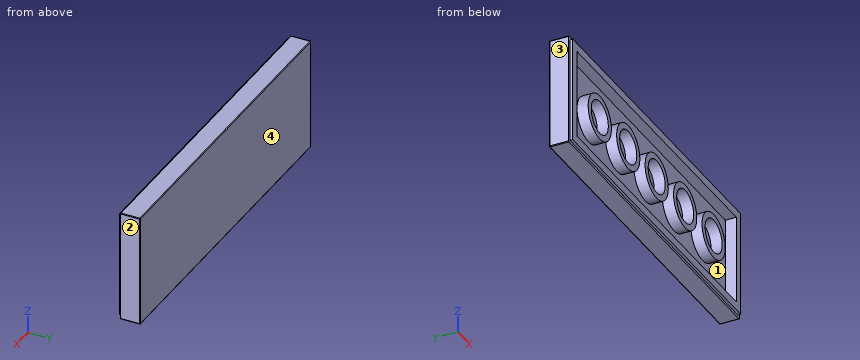
Autodesk Inventor part; units mm, degrees
ref_plane "YZ Plane" through (0, 0, 0) normal (1, 0, 0) x (0, 1, 0)
ref_plane "XZ Plane" through (0, 0, 0) normal (0, 1, 0) x (-1, 0, 0)
ref_plane "XY Plane" through (0, 0, 0) normal (0, 0, 1) x (1, 0, 0)
sketch "Sketch2" plane through (0, 0, 0) normal (0, 1, 0) x (-1, 0, 0)
  line L0 (-24, 8) -> (24, 8)
  line L1 (24, 8) -> (24, -8)
  line L2 (24, -8) -> (-24, -8)
  line L3 (-24, -8) -> (-24, 8)
  point P0 (0, 0)
  point P1 (0, 8)
  point P2 (-24, 0)
  dimension "d0" = 48
  dimension "d1" = 16
extrude "Extrusion1" add sketch "Sketch2" along normal blind 3.2
sketch "Sketch3" plane through (0, 0, 0) normal (0, -1, 0) x (1, 0, 0)
  line L0 (-24, 8) -> (-24, -8)
  line L1 (-22.4, 6.4) -> (22.4, 6.4)
  line L2 (22.4, 6.4) -> (22.4, -6.4)
  line L3 (22.4, -6.4) -> (-22.4, -6.4)
  line L4 (-22.4, -6.4) -> (-22.4, 6.4)
  circle A0 centre (-16, 0) radius 3.2569
  circle A1 centre (-16, 0) radius 2.4
  line L5 (-24, -8) -> (24, -8)
  circle A2 centre (0, 0) radius 1.6
  line L6 (24, -8) -> (24, 8)
  line L7 (-12, 0) -> (-4, 0) construction
  line L8 (-4, 0) -> (4, 0) construction
  line L9 (4, 0) -> (12, 0) construction
  circle A3 centre (-20, 4) radius 2.4 construction
  circle A4 centre (-20, -4) radius 2.4 construction
  circle A5 centre (20, -4) radius 2.4 construction
  circle A6 centre (20, 4) radius 2.4 construction
  line L10 (24, 8) -> (-24, 8)
  line L11 (-23.6, 7.6) -> (23.6, 7.6)
  line L12 (23.6, 7.6) -> (23.6, -7.6)
  line L13 (23.6, -7.6) -> (-23.6, -7.6)
  line L14 (-23.6, -7.6) -> (-23.6, 7.6)
  point P0 (-22.4, 0)
  point P1 (0, 6.4)
  point P2 (0, 0)
  point P3 (0, 7.6)
  point P4 (-23.6, 0)
  dimension "d61" = 4.8
  dimension "d75" = 8
  dimension "d76" = 8
  dimension "d86" = 3.2
  dimension "d92" = 8
  dimension "d98" = 40
  dimension "d99" = 8
  dimension "d102" = 0.4
  dimension "d103" = 0.4
extrude "Extrusion2" cut sketch "Sketch3" against normal blind 1.6 contours L1 L2 L3 L4 | A0 | A1 | A2
extrude "Extrusion7" cut sketch "Sketch3" against normal blind 0.4 contours L10 L6 L5 L0
extrude "Extrusion6" add sketch "Sketch3" against normal up to next contours A0
pattern_linear "Rectangular Pattern3" count 5 spacing 8 along (1, 0, 0) of "Extrusion6"
fillet "Fillet1" radius 0.1 8 edges at (-24, 1.8, 8) (0, 3.2, 8) (-24, 3.2, 0) (0, 3.2, -8) (24, 3.2, 0) (24, 1.8, 8) (24, 1.8, -8) (-24, 1.8, -8)
sketch "Skizze10" plane through (0, 3.2, 0) normal (0, 1, 0) x (1, 0, 0)
  line L0 (-21.913, 4.8) -> (21.913, 4.8) construction
  line L1 (21.913, 4.8) -> (21.913, -4.8) construction
  line L2 (21.913, -4.8) -> (-21.913, -4.8) construction
  line L3 (-21.913, -4.8) -> (-21.913, 4.8) construction
  line L4 (23.9, 8) -> (-23.9, 8)
  line L5 (-23.9, -8) -> (23.9, -8)
  point P0 (0, 0)
  point P1 (0, 4.8)
  point P2 (0, 8)
  dimension "d107" = 3.2
  dimension "d110" = 3.2
decal "Aufkleber1"
equation "\"d4\" = 0.333333 * lh"
equation "\"d61\" = kd"
equation "\"d75\" = lu"
equation "\"d76\" = d75"
equation "\"d86\" = pd"
equation "\"d92\" = lu"
equation "\"d98\" = 5 * lu"
equation "\"d99\" = d75"
equation "\"d102\" = gw"
equation "\"d103\" = gw"
equation "\"d11\" = 0.333333 * lh - topthk"
equation "\"d104\" = gh"
equation "\"d91\" = lu"
equation "\"d110\" = d107"
properties part number "69729-DkBluishGray" material "ABS Plastic"
Check sheet for the modelled part. Datum: model origin and axes. Units: mm. Face numbers are marked on the shaded views. Give positions to 0.01 mm unless a question says otherwise; leave off trailing zeros. Write each loop counter-clockwise with the first axis right and the second up, starting at its lowest first coordinate (ties: lowest second). Pieces come first, ordered by that corner, then holes. Notation, with made-up numbers: (-17.75, 37.5) -> (4.25, 37.5) arc R26 ccw to (4.25, 63.5) -> close; hole circle Ø5 at (48.25, -10.75). An arc over 180 degrees is marked (long way). Use CSV: the item, a comma, the result in double quotes. Start each with the question number.
Q1. Cross-section at C-C on x = 9. Enter the section's corners in (y, z), and give its area (3 significant figures).
Q2. Scan lines: line 1 along Z through (x, y) = (0, 1.25); line 2 along Z through (x, y) = (-1, 0.2); line 3 along Z through (x, y) = (-4.5, 1.45). Record each from-to range of solid material in increasing order.
Q3. Depth check by flat-ended pin: P1, Ø5.5, axis at x = 16.5, z = 0.5, coming from the -Y side; P2, Ø4.5, axis at x = 0, z = 0, coming from the -Y side. Enter the tip coordinate at first touch or a pass-through.
Q4. Cross-section at A-A on x = -8. Enter the section's corners in (y, z).
Q5. Release check for a two-part mould opening along X. For the marked faces 1, 2, 3 and 4 record: +X half, -X half, draft (parallel to the pull), parting line (faces both ways), or undercut.
Q6. Cross-section at B-B on z = 3.75. Enter the section's corners in (x, y), and give its area (3 significant figures).
Working result:
1,outline,"(0, -7.6) -> (0.4, -7.6) -> (0.4, -8) -> (3.1, -8) arc R0.1 ccw to (3.2, -7.9) -> (3.2, 7.9) arc R0.1 ccw to (3.1, 8) -> (0.4, 8) -> (0.4, 7.6) -> (0, 7.6) -> (0, 6.4) -> (1.6, 6.4) -> (1.6, 3.1) -> (0, 3.1) -> (0, 2.18) -> (1.6, 2.18) -> (1.6, -2.18) -> (0, -2.18) -> (0, -3.1) -> (1.6, -3.1) -> (1.6, -6.4) -> (0, -6.4) -> close"
1,area,"33.3 mm^2"
2,line 1,"z = -8 to -6.4, -3.26 to -2.4, 2.4 to 3.26, 6.4 to 8"
2,line 2,"z = -7.6 to -6.4, -3.1 to -2.18, 2.18 to 3.1, 6.4 to 7.6"
2,line 3,"z = -8 to -6.4, 6.4 to 8"
3,P1,"stops at y = 0"
3,P2,"stops at y = 1.6"
4,outline,"(0, -7.6) -> (0.4, -7.6) -> (0.4, -8) -> (3.1, -8) arc R0.1 ccw to (3.2, -7.9) -> (3.2, 7.9) arc R0.1 ccw to (3.1, 8) -> (0.4, 8) -> (0.4, 7.6) -> (0, 7.6) -> (0, 6.4) -> (1.6, 6.4) -> (1.6, 3.26) -> (0, 3.26) -> (0, 2.4) -> (1.6, 2.4) -> (1.6, -2.4) -> (0, -2.4) -> (0, -3.26) -> (1.6, -3.26) -> (1.6, -6.4) -> (0, -6.4) -> close"
5,face 1,"undercut"
5,face 2,"+X half"
5,face 3,"-X half"
5,face 4,"draft"
6,outline,"(-24, 0.4) -> (-23.6, 0.4) -> (-23.6, 0) -> (-22.4, 0) -> (-22.4, 1.6) -> (22.4, 1.6) -> (22.4, 0) -> (23.6, 0) -> (23.6, 0.4) -> (24, 0.4) -> (24, 3.1) arc R0.1 ccw to (23.9, 3.2) -> (-23.9, 3.2) arc R0.1 ccw to (-24, 3.1) -> close"
6,area,"81.6 mm^2"
